```python
from build123d import *

# Parameters (mm, degrees)
ESBO_O9_W                      = 25
ESBO_O9_H                      = 16
FLANGE_BASE2_DEPTH             = 2
ARESTA_FLANGE2_STRIP_W         = 10
ARESTA_FLANGE2_STRIP_H         = 2
ARESTA_FLANGE2_STRIP_CUT_DEPTH = 25
ARESTA_FLANGE2_DEPTH           = 25
ARESTA_FLANGE3_STRIP_W         = 10
ARESTA_FLANGE3_STRIP_H         = 2
ARESTA_FLANGE3_STRIP_CUT_DEPTH = 25
ARESTA_FLANGE3_DEPTH           = 25
FILETE1_R                      = 1
CORTE_EXTRUS_O1_REACH          = 34.016
ESBO_O21_R                     = 1.75
ESBO_O22_R                     = 1.75
CORTE_EXTRUS_O2_DEPTH          = 10


# Sheet-metal steps are written as plain solids
with BuildPart() as part:
    # Esboço9 → Flange-base2 (new body)
    with BuildSketch(Plane.XY):
        with Locations((12.5, 8)):
            Rectangle(ESBO_O9_W, ESBO_O9_H)
    extrude(amount=FLANGE_BASE2_DEPTH)

    # Aresta-Flange2 strip (across the edge) → Aresta-Flange2 strip cut (cut)
    with BuildSketch(Plane(origin=(25, 0, 0), x_dir=(0, 1, 0), z_dir=(-1, 0, 0))):
        with Locations((-2, -1)):
            Rectangle(ARESTA_FLANGE2_STRIP_W, ARESTA_FLANGE2_STRIP_H)
    extrude(amount=ARESTA_FLANGE2_STRIP_CUT_DEPTH, mode=Mode.SUBTRACT)

    # Aresta-Flange2 section (across the edge) → Aresta-Flange2 (add)
    with BuildSketch(Plane(origin=(25, 0, 0), x_dir=(0, 1, 0), z_dir=(-1, 0, 0))):
        with BuildLine():
            Line((0, 1), (0, 10))
            Line((0, 10), (2, 10))
            Line((2, 10), (2, 1))
            ThreePointArc((2, 1), (2.292893219, 0.292893219), (3, 0))
            Line((3, 0), (3, -2))
            ThreePointArc((3, -2), (0.878679656, -1.121320344), (0, 1))
        make_face()
    extrude(amount=ARESTA_FLANGE2_DEPTH)

    # Aresta-Flange3 strip (across the edge) → Aresta-Flange3 strip cut (cut)
    with BuildSketch(Plane(origin=(25, 2, -10), x_dir=(0, 0, 1), z_dir=(-1, 0, 0))):
        with Locations((-2, -1)):
            Rectangle(ARESTA_FLANGE3_STRIP_W, ARESTA_FLANGE3_STRIP_H)
    extrude(amount=ARESTA_FLANGE3_STRIP_CUT_DEPTH, mode=Mode.SUBTRACT)

    # Aresta-Flange3 section (across the edge) → Aresta-Flange3 (add)
    with BuildSketch(Plane(origin=(25, 2, -10), x_dir=(0, 0, 1), z_dir=(-1, 0, 0))):
        with BuildLine():
            Line((0, 1), (0, 14))
            Line((0, 14), (2, 14))
            Line((2, 14), (2, 1))
            ThreePointArc((2, 1), (2.292893219, 0.292893219), (3, 0))
            Line((3, 0), (3, -2))
            ThreePointArc((3, -2), (0.878679656, -1.121320344), (0, 1))
        make_face()
    extrude(amount=ARESTA_FLANGE3_DEPTH)

    # Filete1
    filete1_edges = [part.edges().sort_by_distance(p)[0] for p in [
        (25, 16, -9),
        (0, 16, -9),
        (0, 16, 1),
        (25, 16, 1),
    ]]
    fillet(filete1_edges, radius=FILETE1_R)

    # Corte-extrusão1: up to this face of the body (flat: up to its plane)
    corte_extrus_o1_end = Plane(part.part.faces().sort_by_distance((12.5, 9.491699951, -10))[0])
    # Esboço21 → Corte-extrusão1 (cut, up to the picked face)
    with BuildSketch(Plane.XY.offset(2), mode=Mode.PRIVATE) as corte_extrus_o1_sk1:
        with Locations(Location((3, 12.75, 0), (0, 0, 270))):
            Circle(ESBO_O21_R)
    corte_extrus_o1_tool1 = split(extrude(corte_extrus_o1_sk1.sketch, amount=-CORTE_EXTRUS_O1_REACH, mode=Mode.PRIVATE), bisect_by=corte_extrus_o1_end, keep=Keep.BOTH, mode=Mode.PRIVATE)
    # Esboço21 → Corte-extrusão1 (cut, up to the picked face)
    with BuildSketch(Plane.XY.offset(2), mode=Mode.PRIVATE) as corte_extrus_o1_sk2:
        with Locations(Location((22, 12.75, 0), (0, 0, 270))):
            Circle(ESBO_O21_R)
    corte_extrus_o1_tool2 = split(extrude(corte_extrus_o1_sk2.sketch, amount=-CORTE_EXTRUS_O1_REACH, mode=Mode.PRIVATE), bisect_by=corte_extrus_o1_end, keep=Keep.BOTH, mode=Mode.PRIVATE)
    add(corte_extrus_o1_tool1.solids().sort_by(Axis((3, 12.75, 2), (0, 0, -1)))[0], mode=Mode.SUBTRACT)
    add(corte_extrus_o1_tool2.solids().sort_by(Axis((22, 12.75, 2), (0, 0, -1)))[0], mode=Mode.SUBTRACT)

    # Esboço22 → Corte-extrusão2 (cut)
    with BuildSketch(Plane(origin=(0, 2, 0), x_dir=(1, 0, 0), z_dir=(0, 1, 0))):
        with Locations(Location((4, 4, 0), (0, 0, 270))):
            Circle(ESBO_O22_R)
        with Locations(Location((21, 4, 0), (0, 0, 270))):
            Circle(ESBO_O22_R)
    extrude(amount=-CORTE_EXTRUS_O2_DEPTH, mode=Mode.SUBTRACT)


solid = part.part
```
For this review, take the finished solid that the model builds, in its own axes (mm). A direction names the side the tool comes from. Round coordinates to 2 decimals unless told otherwise and drop trailing zeros. Write each loop counter-clockwise with the first axis right and the second up, starting at its lowest first coordinate (ties: lowest second). Pieces come first, ordered by that corner, then holes.
1) Take a section at C-C on y = 12.75. Give the boundary of the cut face in (x, z), then the cut area to 3 significant figures.
Answer below:
outline: (0, -10) - (1.25, -10) - (1.25, -8) - (0, -8) - close; (0, 0) - (1.25, 0) - (1.25, 2) - (0, 2) - close; (4.75, -10) - (20.25, -10) - (20.25, -8) - (4.75, -8) - close; (4.75, 0) - (20.25, 0) - (20.25, 2) - (4.75, 2) - close; (23.75, -10) - (25, -10) - (25, -8) - (23.75, -8) - close; (23.75, 0) - (25, 0) - (25, 2) - (23.75, 2) - close
area: 72.0 mm2
2) Mouldability with a two-part tool opening along Z and no side actions: class faces 1 (the face through (24.715, 15.699, 1.014)), 2 (the face through (12.68, 0.86, -9.1)), 3 (the face through (13, 10, -8)), 4 (the face through (12.68, 0.9, 1.14)) as +Z half, -Z half, draft (parallel to the pull), parting line (faces both ways), or undercut.
Answer below:
face 1: draft
face 2: -Z half
face 3: undercut
face 4: +Z half
3) Take a section at D-D on x = 4. Give the boundary of the cut face in (y, z), then the cut area to 3 significant figures.
Answer below:
outline: (0, -7) arc R3 ccw to (3, -10) - (11.31, -10) - (11.31, -8) - (3, -8) arc R1 cw to (2, -7) - (2, -5.75) - (0, -5.75) - close; (0, -2.25) - (2, -2.25) - (2, -1) arc R1 cw to (3, 0) - (11.31, 0) - (11.31, 2) - (3, 2) arc R3 ccw to (0, -1) - close; (14.19, -10) - (16, -10) - (16, -8) - (14.19, -8) - close; (14.19, 0) - (16, 0) - (16, 2) - (14.19, 2) - close
area: 58.1 mm2
4) Insertion check: pin 1 Ø4.5 at (x, z) = (4, -4) entering from +Y; pin 2 Ø3 at (x, z) = (15.5, -6) entering from +Y; pin 3 Ø3 at (x, y) = (3, 12.75) entering from -Z. Each pin has a flat end and moves straight along its axis. Give the tip position at first contact, or say it passes through.
Answer below:
pin 1: stops at y = 2
pin 2: stops at y = 2.13
pin 3: passes through
5) Take a section at B-B on z = -4. Give the boundary of the cut face in (x, y).
Answer below:
outline: (0, 0) - (2.25, 0) - (2.25, 2) - (0, 2) - close; (5.75, 0) - (19.25, 0) - (19.25, 2) - (5.75, 2) - close; (22.75, 0) - (25, 0) - (25, 2) - (22.75, 2) - close
6) Take a section at A-A on y = 9.5. Give the boundary of the cut face in (x, z), then the cut area to 3 significant figures.
Answer below:
outline: (0, -10) - (25, -10) - (25, -8) - (0, -8) - close; (0, 0) - (25, 0) - (25, 2) - (0, 2) - close
area: 100 mm2
7) For line 1 along X through (y, z) = (12.75, 1.35); line 2 along Z through (x, y) = (8, 3.75); line 3 along Y through (x, z) = (16.5, -3), list the stretches that pass through material, from the lowest coordinate up.
Answer below:
line 1: x = 0 to 1.25, 4.75 to 20.25, 23.75 to 25
line 2: z = -10 to -8, 0 to 2
line 3: y = 0 to 2
8) Machinability: for faces 5 (the face through (13, 9, -10)), 6 (the face through (12.675, 2.285, -0.301)), which of the approach directions +Z, -Z, +X, -X, +Y, -Y give a long, thin tool a straight path to every point of the face, cutting with its end or side? Answer none if there is none.
Answer below:
face 5: -Z, +X, -X, +Y, -Y
face 6: +X, -X, +Y
